```python
from build123d import *

# Parameters (mm, degrees)
RESSALTO_EXTRUS_O1_DEPTH = 2


with BuildPart() as part:
    # Esboço1 → Ressalto-extrusão1 (new body)
    with BuildSketch(Plane.XY):
        with BuildLine():
            Line((-35, 0), (0, 0))
            Line((0, 0), (35, 0))
            Line((35, 0), (35, 5))
            Line((35, 5), (45, 5))
            Line((45, 5), (45, 13))
            Line((45, 13), (44.031459095, 13))
            Line((44.031459095, 13), (44.031459095, 11))
            ThreePointArc((44.031459095, 11), (43.141182377, 10.109723283), (42.25090566, 11))
            Line((42.25090566, 11), (42.25090566, 13))
            Line((42.25090566, 13), (35, 13))
            Line((35, 13), (35, 20))
            Line((35, 20), (12, 20))
            Line((12, 20), (12, 11))
            ThreePointArc((12, 11), (11, 10), (10, 11))
            Line((10, 11), (10, 20))
            Line((10, 20), (-10, 20))
            Line((-10, 20), (-10, 11))
            ThreePointArc((-10, 11), (-11, 10), (-12, 11))
            Line((-12, 11), (-12, 20))
            Line((-12, 20), (-35, 20))
            Line((-35, 20), (-35, 13))
            Line((-35, 13), (-42.25090566, 13))
            Line((-42.25090566, 13), (-42.25090566, 11))
            ThreePointArc((-42.25090566, 11), (-43.141182377, 10.109723283), (-44.031459095, 11))
            Line((-44.031459095, 11), (-44.031459095, 13))
            Line((-44.031459095, 13), (-45, 13))
            Line((-45, 13), (-45, 5))
            Line((-45, 5), (-35, 5))
            Line((-35, 5), (-35, 0))
        make_face()
    extrude(amount=RESSALTO_EXTRUS_O1_DEPTH)


solid = part.part
```
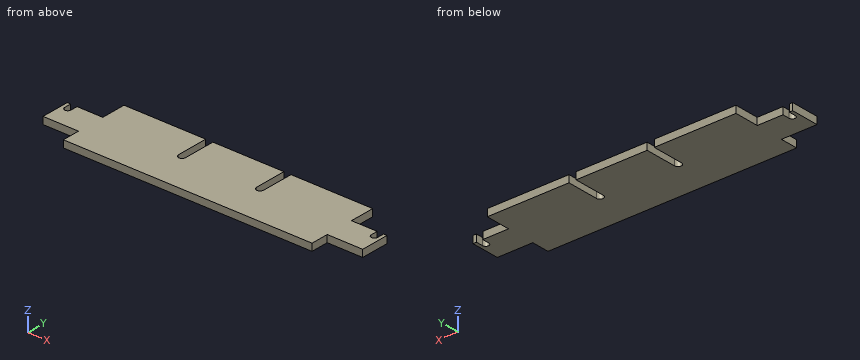
Build history of the part. All positions in model axes, mm. Give positions to 0.01 mm unless a question says otherwise; leave off trailing zeros. Order: outer loops, then holes, each group sorted by start corner. A loop starts at its lowest first (then second) coordinate and runs counter-clockwise, first axis right, second up. Notation, with made-up numbers: M -22.5,25 L 10.5,25 A29 ccw 10.5,59 Z; hole C 70.25,-12 d10. An arc over 180 degrees is marked long. Write item = value, one per line. Start each with the question number.
(1) Pin check, flat tips, straight feed: pin 1 Ø1 at (x, z) = (39, 1) entering from +Y; pin 2 Ø0.6 at (y, z) = (15.5, 0.5) entering from -X; pin 3 Ø1 at (x, z) = (-19.5, 1.5) entering from -Y; pin 4 Ø0.6 at (y, z) = (14, 1) entering from +X. Stop position of each tip, or through.
(2) Slice it at A-A on y = 17.5. Write the cut outline in (x, z), plus the area to 3 significant figures.
(3) Probe L1, parallel to X at y = 19.25, z = 1.55; L2, parallel to X at y = 12.5, z = 0.45; L3, parallel to X at y = 2, z = 1.2. List the from-to ranges inside material, lowest first. Write a range as [from, to].
(4) Slice it at D-D on y = 1.5. Write the cut outline in (x, z).
(5) Slice it at C-C on x = 11. Write the cut outline in (y, z).
(6) Slice it at B-B on z = 0.6. Write the cut outline in (x, y).
Responses:
q1.pin_1 = 13
q1.pin_2 = -35
q1.pin_3 = 0
q1.pin_4 = 35
q2.outline = M -35,0 L -12,0 L -12,2 L -35,2 Z; M -10,0 L 10,0 L 10,2 L -10,2 Z; M 12,0 L 35,0 L 35,2 L 12,2 Z
q2.area = 132 mm2
q3.L1 = [-35, -12], [-10, 10], [12, 35]
q3.L2 = [-45, -44.03], [-42.25, -12], [-10, 10], [12, 42.25], [44.03, 45]
q3.L3 = [-35, 35]
q4.outline = M -35,0 L 35,0 L 35,2 L -35,2 Z
q5.outline = M 0,0 L 10,0 L 10,2 L 0,2 Z
q6.outline = M -45,5 L -35,5 L -35,0 L 35,0 L 35,5 L 45,5 L 45,13 L 44.03,13 L 44.03,11 A0.89 cw 42.25,11 L 42.25,13 L 35,13 L 35,20 L 12,20 L 12,11 A1 cw 10,11 L 10,20 L -10,20 L -10,11 A1 cw -12,11 L -12,20 L -35,20 L -35,13 L -42.25,13 L -42.25,11 A0.89 cw -44.03,11 L -44.03,13 L -45,13 Z
